Build history of the part. All positions in model axes, mm. Give positions to 0.01 mm unless a question says otherwise; leave off trailing zeros. Loops run counter-clockwise (first coordinate to the right, second up) from the corner with the lowest first, then second, coordinate; pieces in that order, holes last. Notation, with made-up numbers: M 45,30 L 72,30 A8 cw 72,42 Z; hole C 24,-37 d5. An arc over 180 degrees is marked long. Put each result on its own line as item: value.
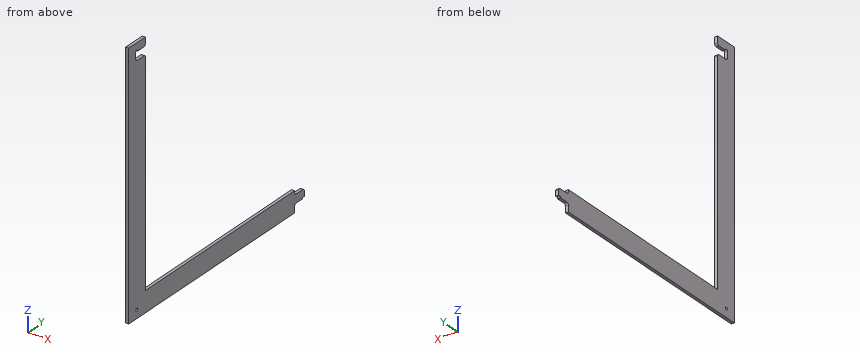
```python
from build123d import *

# Parameters (mm, degrees)
SKETCH2_R           = 2
BOSS_EXTRUDE1_DEPTH = 4.5
CUT_EXTRUDE1_DEPTH  = 517.996374688
FILLET2_R           = 0.5
FILLET4_R           = 0.5
FILLET5_R           = 0.5
FILLET6_R           = 3
FILLET7_R           = 3


with BuildPart() as part:
    # Sketch2 → Boss-Extrude1 (new body)
    # profile 1 of 2: a face of its own
    with BuildSketch(Plane(origin=(0, 0, 0), x_dir=(0, 0, -1), z_dir=(1, 0, 0))):
        Polygon((-12, 339), (0, 339), (0, 0), (-372, 0), (-372, 30), (-360, 30), (-360, 10), (-348, 10), (-348, 30), (-30, 30), (-30, 339), (-24, 339), (-24, 359), (-12, 359), align=None)
        with Locations((-12, 12)):
            Circle(SKETCH2_R, mode=Mode.SUBTRACT)
    # profile 2 of 2: a face of its own
    with BuildSketch(Plane(origin=(0, 0, 0), x_dir=(0, 0, -1), z_dir=(1, 0, 0))):
        Polygon((-372.000001936, -4.49995894), (0, -4.500002581), (0, 0), (-372, 0), align=None)
    extrude(amount=BOSS_EXTRUDE1_DEPTH)

    # Sketch3 → Cut-Extrude1 (cut, through all)
    with BuildSketch(Plane(origin=(0, 0, 0), x_dir=(0, 0, -1), z_dir=(1, 0, 0))):
        with BuildLine():
            Line((-360, 14), (-360, 10))
            ThreePointArc((-360, 10), (-358.585786438, 10.585786438), (-358, 12))
            ThreePointArc((-358, 12), (-358.585786438, 13.414213562), (-360, 14))
        make_face()
        with BuildLine():
            ThreePointArc((-360, 14), (-362, 12), (-360, 10))
            Line((-360, 10), (-360, 14))
        make_face()
        with BuildLine():
            ThreePointArc((-12, 355), (-10.585786438, 355.585786438), (-10, 357))
            ThreePointArc((-10, 357), (-10.585786438, 358.414213562), (-12, 359))
            Line((-12, 359), (-12, 355))
        make_face()
        with BuildLine():
            Line((-12, 355), (-12, 359))
            ThreePointArc((-12, 359), (-14, 357), (-12, 355))
        make_face()
    extrude(amount=CUT_EXTRUDE1_DEPTH, mode=Mode.SUBTRACT)

    # Fillet2
    fillet2_edges = [part.edges().sort_by_distance(p)[0] for p in [
        (2.25, 355, 12),
    ]]
    fillet(fillet2_edges, radius=FILLET2_R)

    # Fillet4
    fillet4_edges = [part.edges().sort_by_distance(p)[0] for p in [
        (2.25, 359, 12),
    ]]
    fillet(fillet4_edges, radius=FILLET4_R)

    # Fillet5
    fillet5_edges = [part.edges().sort_by_distance(p)[0] for p in [
        (2.25, 14, 360),
    ]]
    fillet(fillet5_edges, radius=FILLET5_R)

    # Fillet6
    fillet6_edges = [part.edges().sort_by_distance(p)[0] for p in [
        (2.25, 30, 360),
        (2.25, 30, 348),
        (2.25, 339, 24),
        (2.25, 339, 12),
    ]]
    fillet(fillet6_edges, radius=FILLET6_R)

    # Fillet7
    fillet7_edges = [part.edges().sort_by_distance(p)[0] for p in [
        (2.25, 10, 348),
        (2.25, 359, 24),
    ]]
    fillet(fillet7_edges, radius=FILLET7_R)


solid = part.part
```
Q1. Slice it at A-A (y = 291). List the corners of the cut face in (x, z), and give its area (3 significant figures).
Here are the results:
outline: M 0,0 L 4.5,0 L 4.5,30 L 0,30 Z
area: 135 mm²
Q2. Drop flat-ended pins along their axis: pin 1 Ø1.3 at (x, y) = (2, 20.5) entering from -Z; pin 2 Ø2 at (x, z) = (1.5, 230.5) entering from +Y; pin 3 Ø2 at (x, y) = (1.5, 221) entering from +Z; pin 4 Ø2 at (x, y) = (3.5, 350) entering from -Z. Give the stop position or say it passes through.
Here are the results:
pin 1: z = 0
pin 2: y = 30
pin 3: z = 30
pin 4: z = 12
Q3. Probe line 1 (Y direction, x = 1.3, z = 176); line 2 (Z direction, x = 1.3, y = 234); line 3 (Z direction, x = 3.8, y = 339.5). List the from-to ranges inside material, lowest first. Write a range as from..to.
Here are the results:
line 1: -4.5..30
line 2: 0..30
line 3: 10.66..25.34
Q4. Slice it at B-B (z = 278.5). List the corners of the cut face in (x, y).
Here are the results:
outline: M 0,-4.5 L 4.5,-4.5 L 4.5,30 L 0,30 Z
